Work out the finished part from the listing and answer in its coordinate system (mm). Face numbers are marked on the shaded views. A direction names the side the tool comes from. Give positions to 0.01 mm unless a question says otherwise; leave off trailing zeros. Loops run counter-clockwise (first coordinate to the right, second up) from the corner with the lowest first, then second, coordinate; pieces in that order, holes last. Notation, with made-up numbers: M 83,76.5 L 129,76.5 A18 cw 129,110.5 Z; hole C 52,20 d10. An arc over 180 degrees is marked long. Answer in a Markdown table with one row per item. Add a question column.
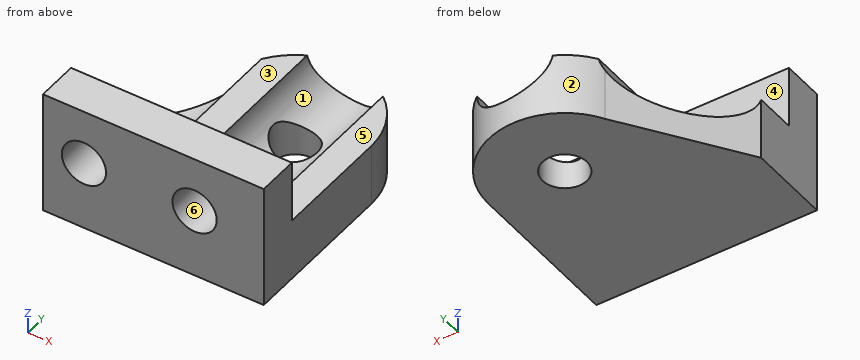
Autodesk Inventor part; units mm, degrees
ref_plane "YZ Plane" through (0, 0, 0) normal (1, 0, 0) x (0, 1, 0)
ref_plane "XZ Plane" through (0, 0, 0) normal (0, 1, 0) x (-1, 0, 0)
ref_plane "XY Plane" through (0, 0, 0) normal (0, 0, 1) x (1, 0, 0)
sketch "Sketch1" plane through (0, 0, 0) normal (0, 0, 1) x (1, 0, 0)
  circle A0 centre (12.5, 11.5) radius 1.6
  line L0 (0, 0) -> (18, 0)
  line L1 (0, 0) -> (0, 3)
  arc A1 (18, 11.5) -> (7.7369, 14.25) centre (12.5, 11.5) ccw
  line L2 (12.5, 11.5) -> (7.7369, 14.25) construction
  line L3 (12.5, 11.5) -> (18, 11.5) construction
  line L4 (7.7369, 14.25) -> (0, 3)
  line L5 (18, 11.5) -> (18, 0)
  dimension "d17" = 3
  dimension "d19" = 11.5
  dimension "d23" = 90
  dimension "d25" = 12.5
  dimension "d31" = 5.5
  dimension "d32" = 150
  dimension "d49" = 3.2
extrude "Extrusion1" add sketch "Sketch1" along normal blind 4.5
sketch "Sketch4" plane through (0, 0, 4.5) normal (0, 0, 1) x (1, 0, 0)
  line L0 (0, 3) -> (0, 0)
  line L1 (18, 0) -> (18, 3)
  line L2 (0, 0) -> (18, 0)
  line L3 (18, 0) -> (18, 3)
  line L4 (18, 3) -> (0, 3)
  line L5 (0, 3) -> (0, 0)
  line L6 (18, 0) -> (18, 11.5)
extrude "Extrusion2" add sketch "Sketch4" along normal blind 4.5
sketch "Sketch5" plane through (0, 0, 0) normal (0, -1, 0) x (1, 0, 0)
  circle A0 centre (5, 5) radius 1.6
  circle A1 centre (13, 5) radius 1.6
  line L0 (0, 0) -> (18, 0)
  point P0 (20.0001, 0)
  dimension "d13" = 3.2
  dimension "d14" = 3.2
  dimension "d38" = 5
  dimension "d39" = 5
  dimension "d50" = 8
extrude "Extrusion3" cut sketch "Sketch5" against normal through all
sketch "Sketch6" plane through (0, 3, 9) normal (0, 1, 0) x (1, 0, 0)
  circle A0 centre (5, 4) radius 1.6
  circle A1 centre (5, 4) radius 3
  circle A2 centre (13, 4) radius 1.6
  circle A3 centre (13, 4) radius 3
  line L0 (0, 9) -> (18, 9)
  point P0 (20.0001, 9)
  dimension "d34" = 6
  dimension "d35" = 6
  dimension "d40" = 5
  dimension "d41" = 5
extrude "Extrusion4" cut sketch "Sketch6" along normal up to next
sketch "Sketch7" plane through (0, 0, 0) normal (0, -1, 0) x (1, 0, 0)
  line L0 (0, 0) -> (0, 9)
  line L1 (2.042, 0) -> (0, 0)
  line L2 (0, 0) -> (0, 9)
  line L3 (0, 9) -> (2.042, 9)
  line L4 (2.042, 9) -> (2.042, 0)
extrude "Extrusion5" cut sketch "Sketch7" against normal up to next
properties part number "lower_deck_shaft_mount_v4_for_AD"
(1) Consider line 1 along Z through (x, y) = (13, 1); line 2 along Y through (x, z) = (8.25, 6); line 3 along Z through (x, y) = (17.5, 11.25). Determine where each line is inside the solid, lowest interval first. Write a range as from..to.
(2) Section B-B, the plane x = 6 is taken. Determine the outline of the cut face in (y, z), and give its area (3 significant figures).
(3) Each of these flat-tipped pins is pushed along its axis until it touches: P1, Ø3.5, axis at x = 10, z = 7, coming from the +Y side; P2, Ø3, axis at x = 5, z = 5, coming from the -Y side; P3, Ø1.7, axis at x = 8.5, y = 12, coming from the +Z side. Where does it stop, or does it pass through?
(4) Section A-A, the plane z = 5 is taken. Determine the outline of the cut face in (x, y).
(5) Section C-C, the plane y = 2.25 is taken. Determine the outline of the cut face in (x, z).
(6) Which of the six approach directions +Z, -Z, +X, -X, +Y, -Y give full straight-line access (tool end or side, diameter ignored) to the marked faces 4, 5 and 6?
(7) The mould has two halves that part along X. Classify the marked faces 1, 2 and 3: pulls with the +X half, pulls with the -X half, needs draft (parallel to the pull), parting line crosses it, or undercut.
(8) Section D-D, the plane z = 1.25 is taken. Determine the outline of the cut face in (x, y).
Numbers:
| question | item | result |
|---|---|---|
| 1 | line 1 | z = 0..3.4, 6.6..9 |
| 1 | line 2 | y = 0..3 |
| 1 | line 3 | z = 0..4.5 |
| 2 | outline | M 0,0 L 11.72,0 L 11.72,2.17 L 3,2.17 L 3,3.75 L 0,3.75 Z; M 0,6.25 L 3,6.25 L 3,9 L 0,9 Z |
| 2 | area | 38.5 mm² |
| 3 | P1 | stops at y = 3 |
| 3 | P2 | passes through |
| 3 | P3 | stops at z = 4.5 |
| 4 | outline | M 2.04,0 L 3.4,0 L 3.4,3 L 2.04,3 Z; M 6.6,0 L 11.4,0 L 11.4,3 L 6.6,3 Z; M 14.6,0 L 18,0 L 18,3 L 14.6,3 Z |
| 5 | outline | M 2.04,0 L 18,0 L 18,9 L 2.04,9 Z; hole C 5,5 d3.2; hole C 13,5 d3.2 |
| 6 | face 4 | +Z, +Y |
| 6 | face 5 | +Z, +X, -X, +Y |
| 6 | face 6 | +Y, -Y |
| 7 | face 1 | undercut |
| 7 | face 2 | parting line crosses it |
| 7 | face 3 | needs draft |
| 8 | outline | M 2.04,0 L 18,0 L 18,11.5 A5.5 ccw 7.74,14.25 L 2.04,5.97 Z; hole C 12.5,11.5 d3.2 |
